Read the model definition and answer for the solid it produces. Units are mm, in the model's axes. Face numbers are marked on the shaded views. A direction names the side the tool comes from. Coordinates: 2 decimals unless noted, no trailing zeros. Order: outer loops, then holes, each group sorted by start corner. A loop starts at its lowest first (then second) coordinate and runs counter-clockwise, first axis right, second up.
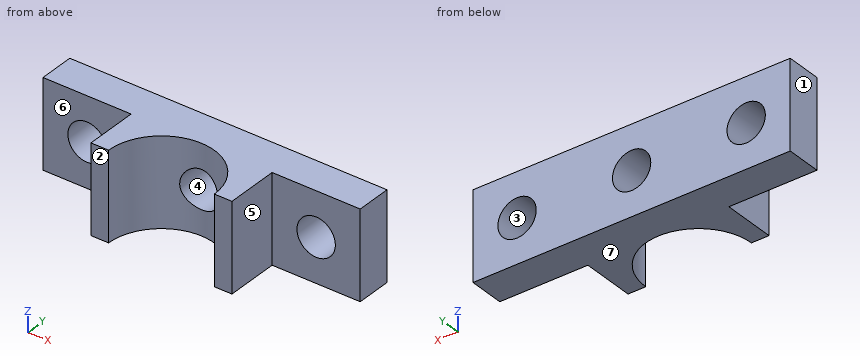
```python
from build123d import *

# Parameters (mm, degrees)
F1_DEPTH = 7.9375
F2_R     = 1.7272
F3_DEPTH = 7.9375


with BuildPart() as f1:
    # F0 (on Top) → F1 (new body)
    with BuildSketch(Plane.XY):
        with BuildLine():
            ThreePointArc((0, 0), (4.7625, 4.7625), (9.525, 0))
            Line((9.525, 0), (11.1125, 0))
            Line((11.1125, 0), (11.1125, 4.7625))
            Line((11.1125, 4.7625), (19.05, 4.7625))
            Line((19.05, 4.7625), (19.05, 7.9375))
            Line((19.05, 7.9375), (-9.525, 7.9375))
            Line((-9.525, 7.9375), (-9.525, 4.7625))
            Line((-9.525, 4.7625), (-1.5875, 4.7625))
            Line((-1.5875, 4.7625), (-1.5875, 0))
            Line((-1.5875, 0), (0, 0))
        make_face()
    extrude(amount=F1_DEPTH)

    # F2 (on face) → F3 (cut, through all)
    with BuildSketch(Plane(origin=(0, 7.9375, 0), x_dir=(-1, 0, 0), z_dir=(0, 1, 0))):
        with Locations((5.55625, 3.96875)):
            Circle(F2_R)
        with Locations((-15.08125, 3.96875)):
            Circle(F2_R)
        with Locations((-4.7625, 3.96875)):
            Circle(F2_R)
    extrude(amount=-F3_DEPTH, mode=Mode.SUBTRACT)


solid = f1.part
```
1) Which of the six approach directions +Z, -Z, +X, -X, +Y, -Y give full straight-line access (tool end or side, diameter ignored) to the marked faces 5, 6 and 7?
A:
face 5: +Z, -Z, +X, -Y
face 6: +Z, -Z, -X, -Y
face 7: -Z, +X, -X, +Y, -Y
2) A cutting plane is placed at A-A, the plane z = 5. State how many separate pieces and enclosed holes the cut face has, and give its area (3 significant figures).
A:
separate pieces: 4
enclosed holes: 0
area: 89.0 mm2
3) Flat-ended cylindrical pins translate along their axes: pin 1 Ø1.5 at (y, z) = (3, 2.5) entering from +X; pin 2 Ø4 at (y, z) = (1.5, 2.5) entering from -X; pin 3 Ø4 at (x, z) = (15.5, 5) entering from -Y. Find the tip coordinate at first contact, or state that the pin passes through.
A:
pin 1: stops at x = 11.11
pin 2: stops at x = -1.59
pin 3: stops at y = 4.76
4) A cutting plane is placed at B-B, the plane x = -5.5. Determine the outline of the cut face in (y, z).
A:
outline: (4.76, 0) - (7.94, 0) - (7.94, 2.24) - (4.76, 2.24) - close; (4.76, 5.7) - (7.94, 5.7) - (7.94, 7.94) - (4.76, 7.94) - close
5) Straight lines are drawn through the part: line 1 (X direction, y = 6, z = 4.5) (3 decimals); line 2 (X direction, y = 6.25, z = 2.75) (3 decimals); line 3 (X direction, y = 2.75, z = 4.25). For each, find the intervals that lie inside material, in ascending order.
A:
line 1: x = -9.525 to -7.2, -3.913 to 3.119, 6.406 to 13.438, 16.725 to 19.05
line 2: x = -9.525 to -6.78, -4.332 to 3.539, 5.986 to 13.857, 16.305 to 19.05
line 3: x = -1.59 to 0.87, 8.65 to 11.11
6) A cutting plane is placed at D-D, the plane y = 3.75. Determine the outline of the cut face in (x, z), and give its area (3 significant figures).
A:
outline: (-1.59, 0) - (1.83, 0) - (1.83, 7.94) - (-1.59, 7.94) - close; (7.7, 0) - (11.11, 0) - (11.11, 7.94) - (7.7, 7.94) - close
area: 54.2 mm2
7) Determine the mould class of the marked faces 1, 2, 3 and 4 for opening direction X: pulls with the +X half, pulls with the -X half, needs draft (parallel to the pull), parting line crosses it, or undercut.
A:
face 1: pulls with the -X half
face 2: needs draft
face 3: undercut
face 4: undercut
